The model under review builds one solid part; all positions refer to its coordinate system, in mm. A direction names the side the tool comes from. Give positions to 0.01 mm unless a question says otherwise; leave off trailing zeros. Loops run counter-clockwise (first coordinate to the right, second up) from the corner with the lowest first, then second, coordinate; pieces in that order, holes last. Notation, with made-up numbers: (-35.75, 15) - (-18.75, 15) arc R29 ccw to (-18.75, 53) - close; hole circle Ø5 at (12.5, 47). An arc over 180 degrees is marked (long way). Answer as a JSON object with one key per item and string values.
from build123d import *

# Parameters (mm, degrees)
BOSS_EXTRUDE1_DEPTH = 19.05


with BuildPart() as part:
    # Sketch1 → Boss-Extrude1 (new body, symmetric)
    with BuildSketch(Plane.XY):
        with BuildLine():
            Line((0, 0), (0, 76.2))
            Line((0, 76.2), (38.0492, 76.2))
            Line((38.0492, 76.2), (38.0492, 74.042335136))
            ThreePointArc((38.0492, 74.042335136), (37.447280466, 72.400554363), (35.926803066, 71.536899509))
            Line((35.926803066, 71.536899509), (12.283671721, 67.596090157))
            ThreePointArc((12.283671721, 67.596090157), (8.178382741, 65.264222052), (6.5532, 60.831413966))
            Line((6.5532, 60.831413966), (6.5532, 15.368586034))
            ThreePointArc((6.5532, 15.368586034), (8.178382741, 10.935777948), (12.283671721, 8.603909843))
            Line((12.283671721, 8.603909843), (35.926803066, 4.663100491))
            ThreePointArc((35.926803066, 4.663100491), (37.447280466, 3.799445637), (38.0492, 2.157664864))
            Line((38.0492, 2.157664864), (38.0492, 0))
            Line((38.0492, 0), (0, 0))
        make_face()
    extrude(amount=BOSS_EXTRUDE1_DEPTH, both=True)


solid = part.part
Q1. Consider section D-D, the plane x = 20.5. State the section outline as (y, z) points.
Results:
{"outline": "(0, -19.05) - (7.23, -19.05) - (7.23, 19.05) - (0, 19.05) - close; (68.97, -19.05) - (76.2, -19.05) - (76.2, 19.05) - (68.97, 19.05) - close"}
Q2. For faces 1 (the face through (19, 76.2, 0)), 2 (the face through (6.553, 38, 0)), list the 3-axis set-ups (+Z, -Z, +X, -X, +Y, -Y) from which the entire face can be reached by the end or side of a thin tool; tool diameter is ignored.
Results:
{"face 1": "+Z, -Z, +X, -X, +Y", "face 2": "+Z, -Z, +X"}
Q3. Consider section C-C, the plane y = 57. State the section outline as (x, z) points, plus the area to 3 significant figures.
Results:
{"outline": "(0, -19.05) - (6.55, -19.05) - (6.55, 19.05) - (0, 19.05) - close", "area": "250 mm^2"}
Q4. To check wall thickness, follow probe 1 along X at (y, z) = (34.5, -12.5); probe 2 along Y at (x, z) = (10.5, -5.5); probe 3 along Y at (x, z) = (32.5, 2). State the ranges of each line that lie inside material, in increasing order. Write a range as [from, to].
Results:
{"probe 1": "x = [0, 6.55]", "probe 2": "y = [0, 9.16], [67.04, 76.2]", "probe 3": "y = [0, 5.23], [70.97, 76.2]"}
Q5. Consider section A-A, the plane x = 14.5. State the section outline as (y, z) points.
Results:
{"outline": "(0, -19.05) - (8.23, -19.05) - (8.23, 19.05) - (0, 19.05) - close; (67.97, -19.05) - (76.2, -19.05) - (76.2, 19.05) - (67.97, 19.05) - close"}
Q6. Consider section B-B, the plane z = -5.5. State the section outline as (x, y) points, plus the area to 3 significant figures.
Results:
{"outline": "(0, 0) - (38.05, 0) - (38.05, 2.16) arc R2.54 ccw to (35.93, 4.66) - (12.28, 8.6) arc R6.86 cw to (6.55, 15.37) - (6.55, 60.83) arc R6.86 cw to (12.28, 67.6) - (35.93, 71.54) arc R2.54 ccw to (38.05, 74.04) - (38.05, 76.2) - (0, 76.2) - close", "area": "948 mm^2"}
Q7. Clearance check with flat-ended pins moving along their axes: pin 1 Ø6 at (x, y) = (24.5, 66) entering from -Z; pin 2 Ø8 at (y, z) = (39, 11.5) entering from +X. State where each tip first meets the part, or that it passes through.
Results:
{"pin 1": "passes through", "pin 2": "stops at x = 6.55"}
Q8. The part is to be moulded in two halves that separate along Y. For faces 3 (the face through (19, 0, 0)), 4 (the face through (24.3, 69.6, 0.3)), 5 (the face through (38.049, 1, 0)), 6 (the face through (8.135, 10.987, 0.267)), say which applies: +Y half, -Y half, draft (parallel to the pull), parting line (faces both ways), or undercut.
Results:
{"face 3": "-Y half", "face 4": "undercut", "face 5": "draft", "face 6": "undercut"}
